```python
from build123d import *

# Parameters (mm, degrees)
SKETCH5_W                      = 100
SKETCH5_H                      = 170
BOSS_EXTRUDE2_DEPTH            = 1
CONVERT_SOLID1_START           = -50
CONVERT_SOLID1_OUTLINE_W       = 170
CONVERT_SOLID1_OUTLINE_H       = 2
CONVERT_SOLID1_DEPTH           = 100
CSK_FOR_M4_SFHCS1_AT_2_COUNT   = 2
CSK_FOR_M4_SFHCS1_AT_2_PITCH   = 15
EDGE_FLANGE3_STRIP_W           = 18
EDGE_FLANGE3_STRIP_H           = 3
EDGE_FLANGE3_STRIP_CUT_DEPTH   = 170
EDGE_FLANGE3_STRIP_2_W         = 18
EDGE_FLANGE3_STRIP_2_H         = 3
EDGE_FLANGE3_STRIP_CUT_2_DEPTH = 170
EDGE_FLANGE3_DEPTH             = 170
EDGE_FLANGE3_BEND_DEPTH        = 170
EDGE_FLANGE4_DEPTH             = 94
EDGE_FLANGE4_BEND_DEPTH        = 94
FILLET1_R                      = 5


# Read off the part's stored shape, not the designer's step: Convert-Solid1
# Sheet-metal steps are written as plain solids
with BuildPart() as part:
    # Sketch5 → Boss-Extrude2 (new body)
    with BuildSketch(Plane.XY):
        Rectangle(SKETCH5_W, SKETCH5_H)
    extrude(amount=BOSS_EXTRUDE2_DEPTH)

    # Convert-Solid1 outline → Convert-Solid1 (add)
    with BuildSketch(Plane.YZ.offset(CONVERT_SOLID1_START)):
        with Locations((0, -1)):
            Rectangle(CONVERT_SOLID1_OUTLINE_W, CONVERT_SOLID1_OUTLINE_H)
    extrude(amount=CONVERT_SOLID1_DEPTH)

    # Sketch23 → CSK for M4 SFHCS1 (revolve, cut)
    with BuildSketch(Plane(origin=(0, -7.5, 1), x_dir=(0, -1, 0), z_dir=(1, 0, 0))):
        Polygon((0, 0), (0, 3), (2.25, 3), (2.25, 2.23), (4.48, 0), align=None)
    csk_for_m4_sfhcs1 = revolve(axis=Axis((0, -7.5, 7.35), (0, 0, -1)), mode=Mode.SUBTRACT)

    # CSK for M4 SFHCS1 at 2: CSK for M4 SFHCS1 ×2
    with Locations(*[(0, i * CSK_FOR_M4_SFHCS1_AT_2_PITCH, 0) for i in range(1, CSK_FOR_M4_SFHCS1_AT_2_COUNT)]):
        add(csk_for_m4_sfhcs1, mode=Mode.SUBTRACT)

    # Edge-Flange3 strip (across the edge) → Edge-Flange3 strip cut (cut)
    with BuildSketch(Plane(origin=(50, -85, 1), x_dir=(-1, 0, 0), z_dir=(0, 1, 0))):
        with Locations((-6, -1.5)):
            Rectangle(EDGE_FLANGE3_STRIP_W, EDGE_FLANGE3_STRIP_H)
    extrude(amount=EDGE_FLANGE3_STRIP_CUT_DEPTH, mode=Mode.SUBTRACT)

    # Edge-Flange3 strip 2 (across the edge) → Edge-Flange3 strip cut 2 (cut)
    with BuildSketch(Plane(origin=(-50, 85, 1), x_dir=(1, 0, 0), z_dir=(0, -1, 0))):
        with Locations((-6, -1.5)):
            Rectangle(EDGE_FLANGE3_STRIP_2_W, EDGE_FLANGE3_STRIP_2_H)
    extrude(amount=EDGE_FLANGE3_STRIP_CUT_2_DEPTH, mode=Mode.SUBTRACT)

    # Edge-Flange3 section (across the edge) → Edge-Flange3 (add)
    with BuildSketch(Plane(origin=(50, -85, 1), x_dir=(-1, 0, 0), z_dir=(0, 1, 0))):
        with BuildLine():
            Line((-3, 3), (-3, 7))
            Line((-3, 7), (0, 7))
            Line((0, 7), (0, 3))
            ThreePointArc((0, 3), (0.878679656, 0.878679656), (3, 0))
            Line((3, 0), (3, -3))
            ThreePointArc((3, -3), (-1.242640687, -1.242640687), (-3, 3))
        make_face()
    extrude(amount=EDGE_FLANGE3_DEPTH)

    # Edge-Flange3 section 2 (across the edge) → Edge-Flange3 bend (add)
    with BuildSketch(Plane(origin=(-50, 85, 1), x_dir=(1, 0, 0), z_dir=(0, -1, 0))):
        with BuildLine():
            Line((-3, 3), (-3, 7))
            Line((-3, 7), (0, 7))
            Line((0, 7), (0, 3))
            ThreePointArc((0, 3), (0.878679656, 0.878679656), (3, 0))
            Line((3, 0), (3, -3))
            ThreePointArc((3, -3), (-1.242640687, -1.242640687), (-3, 3))
        make_face()
    extrude(amount=EDGE_FLANGE3_BEND_DEPTH)

    # Edge-Flange4 section (across the edge) → Edge-Flange4 (add)
    with BuildSketch(Plane(origin=(47, -88, -2), x_dir=(0, 1, 0), z_dir=(-1, 0, 0))):
        with BuildLine():
            Line((-3, 3), (-3, 7))
            Line((-3, 7), (0, 7))
            Line((0, 7), (0, 3))
            ThreePointArc((0, 3), (0.878679656, 0.878679656), (3, 0))
            Line((3, 0), (3, -3))
            ThreePointArc((3, -3), (-1.242640687, -1.242640687), (-3, 3))
        make_face()
    extrude(amount=EDGE_FLANGE4_DEPTH)

    # Edge-Flange4 section 2 (across the edge) → Edge-Flange4 bend (add)
    with BuildSketch(Plane(origin=(-47, 88, -2), x_dir=(0, -1, 0), z_dir=(1, 0, 0))):
        with BuildLine():
            Line((-3, 3), (-3, 7))
            Line((-3, 7), (0, 7))
            Line((0, 7), (0, 3))
            ThreePointArc((0, 3), (0.878679656, 0.878679656), (3, 0))
            Line((3, 0), (3, -3))
            ThreePointArc((3, -3), (-1.242640687, -1.242640687), (-3, 3))
        make_face()
    extrude(amount=EDGE_FLANGE4_BEND_DEPTH)

    # Fillet1
    fillet1_edges = [part.edges().sort_by_distance(p)[0] for p in [
        (51.5, -85, 8),
        (51.5, 85, 8),
        (47, 89.5, -9),
        (-47, 89.5, -9),
        (-51.5, 85, 8),
        (-51.5, -85, 8),
        (-47, -89.5, -9),
        (47, -89.5, -9),
    ]]
    fillet(fillet1_edges, radius=FILLET1_R)


solid = part.part
```
CAD build for the part. Positions are in the model's coordinates, mm. A direction names the side the tool comes from. Round coordinates to 2 decimals unless told otherwise and drop trailing zeros. Write each loop counter-clockwise with the first axis right and the second up, starting at its lowest first coordinate (ties: lowest second). Pieces come first, ordered by that corner, then holes. Notation, with made-up numbers: (69, 46) - (125, 46) arc R26 cw to (125, 72) - close; hole circle Ø3 at (61.5, 23.25). An arc over 180 degrees is marked (long way). Write item = value, one per line. Start each with the question number.
Q1. Drop flat-ended pins along their axis: pin 1 (6 mm diameter, centred on x = 0, y = 7.5, fed in from -Z); pin 2 (3 mm diameter, centred on x = -12.5, y = -60, fed in from +Z); pin 3 (2.5 mm diameter, centred on x = -50.5, z = 1.5, fed in from +Y); pin 4 (4 mm diameter, centred on x = 0, y = -7.5, fed in from -Z). Give the stop position or say it passes through.
Q2. Band-saw the part on A-A (y = 7.5). Give the cut face in (x, z).
Q3. Which spindle directions (+Z, -Z, +X, -X, +Y, -Y) get a long thin tool onto all of the face, cutting with end or side? Do faces 4 (the flat face through (-50, -85, 1)), 5 (the flat face through (50, -85, 1)), 6 (the flat face through (1, -88, -7)), 7 (the flat face through (-1, 1, 1)), 8 (the flat face through (-50, 85, 1)). Say none if no direction does.
Q4. Mould opens along Y. For faces 1 (the cylindrical face through (-0.658, 89.196, -0.711)), 2 (the flat face through (-1, -1, -2)), 3 (the cylindrical face through (0.658, -89.196, -0.711)) say: pulls with the +Y half, pulls with the -Y half, needs draft (parallel to the pull), parting line crosses it, or undercut.
Q5. Band-saw the part on C-C (z = -7.25). Give the cut face in (x, y), then the cut area to 3 significant figures.
Q6. Band-saw the part on B-B (x = 0). Give the cut face in (y, z).
Q7. Band-saw the part on D-D (y = 66.5). Give the cut face in (x, z), then the cut area to 3 significant figures.
Q8. Probe L1, parallel to Y at x = 0, z = -1.8; L2, parallel to Y at x = 0, z = -1.7; L3, parallel to Y at x = 22, z = -8.25. List the from-to ranges inside material, lowest first. Write a range as from..to.
Answers below:
q1.pin_1 = -2
q1.pin_2 = 1
q1.pin_3 = 85
q1.pin_4 = through
q2.outline = (-53, 4) arc R6 ccw to (-47, -2) - (-2.25, -2) - (-2.25, -1.23) - (-4.48, 1) - (-47, 1) arc R3 cw to (-50, 4) - (-50, 8) - (-53, 8) - close; (2.25, -2) - (47, -2) arc R6 ccw to (53, 4) - (53, 8) - (50, 8) - (50, 4) arc R3 cw to (47, 1) - (4.48, 1) - (2.25, -1.23) - close
q3.face_4 = +Z, -Z, -X, -Y
q3.face_5 = +Z, -Z, +X, -Y
q3.face_6 = -Z, +X, -X
q3.face_7 = +Z, +Y, -Y
q3.face_8 = +Z, -Z, -X, +Y
q4.face_1 = pulls with the +Y half
q4.face_2 = undercut
q4.face_3 = pulls with the -Y half
q5.outline = (-45.8, -91) - (45.8, -91) - (45.8, -88) - (-45.8, -88) - close; (-45.8, 88) - (45.8, 88) - (45.8, 91) - (-45.8, 91) - close
q5.area = 550 mm2
q6.outline = (-91, -9) - (-88, -9) - (-88, -5) arc R3 cw to (-85, -2) - (-9.75, -2) - (-9.75, -1.23) - (-11.98, 1) - (-85, 1) arc R6 ccw to (-91, -5) - close; (-5.25, -2) - (5.25, -2) - (5.25, -1.23) - (3.02, 1) - (-3.02, 1) - (-5.25, -1.23) - close; (9.75, -2) - (85, -2) arc R3 cw to (88, -5) - (88, -9) - (91, -9) - (91, -5) arc R6 ccw to (85, 1) - (11.98, 1) - (9.75, -1.23) - close
q7.outline = (-53, 4) arc R6 ccw to (-47, -2) - (47, -2) arc R6 ccw to (53, 4) - (53, 8) - (50, 8) - (50, 4) arc R3 cw to (47, 1) - (-47, 1) arc R3 cw to (-50, 4) - (-50, 8) - (-53, 8) - close
q7.area = 348 mm2
q8.L1 = -90.08..-9.75, -5.25..5.25, 9.75..90.08
q8.L2 = -90.01..-9.75, -5.25..5.25, 9.75..90.01
q8.L3 = -91..-88, 88..91
